```python
from build123d import *

# Parameters (mm, degrees)
SKETCH1_R                                       = 5
SKETCH1_R_2                                     = 1.6
SKETCH1_R_3                                     = 1.25
SKETCH1_R_4                                     = 1.55
BOSS_EXTRUDE1_DEPTH                             = 3.18
CSK_FOR_M2_FLAT_HEAD_MACHINE_SCREW1_D           = 2.4
CSK_FOR_M2_FLAT_HEAD_MACHINE_SCREW1_DEPTH       = 3.508967257
CSK_FOR_M2_FLAT_HEAD_MACHINE_SCREW1_CSINK_D     = 4.4
CSK_FOR_M2_FLAT_HEAD_MACHINE_SCREW1_CSINK_ANGLE = 90
CSK_FOR_M2_FLAT_HEAD_MACHINE_SCREW1_TIP         = 0.721032743
SKETCH3_R                                       = 5
CUT_EXTRUDE4_DEPTH                              = 67.382158748
FILLET2_R                                       = 3
CHAMFER2_SIZE                                   = 1.8


with BuildPart() as part:
    # Sketch1 → Boss-Extrude1 (new body)
    with BuildSketch(Plane(origin=(0, 0, 0), x_dir=(0, 0, -1), z_dir=(1, 0, 0))):
        Polygon((0, 0), (0, 30.2), (2, 32.2), (2, 61.31), (22, 61.31), (22, 41.31), (23.8, 41.31), (23.8, 24.71), (15.9, 24.71), (15.9, 13.26), (13.4, 13.26), (13.4, 11.86), (25.25, 11.86), (25.25, 6.86), (13.4, 6.86), (13.4, 0), align=None)
        with Locations(Location((7, 25.2, 0), (0, 0, 180))):
            Circle(SKETCH1_R, mode=Mode.SUBTRACT)
        with Locations(Location((7, 56.81, 0), (0, 0, 180))):
            Circle(SKETCH1_R_2, mode=Mode.SUBTRACT)
        with Locations(Location((17, 54.81, 0), (0, 0, 180))):
            Circle(SKETCH1_R_2, mode=Mode.SUBTRACT)
        with Locations(Location((22.4, 9.36, 0), (0, 0, 180))):
            Circle(SKETCH1_R_3, mode=Mode.SUBTRACT)
        with Locations(Location((16.4, 9.36, 0), (0, 0, 180))):
            Circle(SKETCH1_R_3, mode=Mode.SUBTRACT)
        with Locations(Location((2.55, 2.55, 0), (0, 0, 180))):
            Circle(SKETCH1_R_4, mode=Mode.SUBTRACT)
        with Locations(Location((2.55, 8.55, 0), (0, 0, 180))):
            Circle(SKETCH1_R_4, mode=Mode.SUBTRACT)
    extrude(amount=BOSS_EXTRUDE1_DEPTH)

    # CSK for M2 Flat Head Machine Screw1
    with Locations(Plane.ZY):
        with Locations((-6.974936087, 46.414674329), (-17.432559713, 42.244769284), (-8.592504199, 35.273154083)):
            CounterSinkHole(CSK_FOR_M2_FLAT_HEAD_MACHINE_SCREW1_D / 2, CSK_FOR_M2_FLAT_HEAD_MACHINE_SCREW1_CSINK_D / 2, depth=CSK_FOR_M2_FLAT_HEAD_MACHINE_SCREW1_DEPTH, counter_sink_angle=CSK_FOR_M2_FLAT_HEAD_MACHINE_SCREW1_CSINK_ANGLE)
            with Locations((0, 0, -(CSK_FOR_M2_FLAT_HEAD_MACHINE_SCREW1_DEPTH + CSK_FOR_M2_FLAT_HEAD_MACHINE_SCREW1_TIP / 2))):  # 118° drill point
                Cone(0, CSK_FOR_M2_FLAT_HEAD_MACHINE_SCREW1_D / 2, CSK_FOR_M2_FLAT_HEAD_MACHINE_SCREW1_TIP, mode=Mode.SUBTRACT)

    # Sketch3 → Cut-Extrude4 (cut, through all)
    with BuildSketch(Plane.ZY):
        with Locations((-11, 41.310865899)):
            Circle(SKETCH3_R)
    extrude(amount=-CUT_EXTRUDE4_DEPTH, mode=Mode.SUBTRACT)

    # Fillet2
    fillet2_edges = [part.edges().sort_by_distance(p)[0] for p in [
        (1.59, 30.2, 0),
        (1.59, 32.2, -2),
    ]]
    fillet(fillet2_edges, radius=FILLET2_R)

    # Chamfer2
    chamfer2_edges = [part.edges().sort_by_distance(p)[0] for p in [
        (1.59, 61.31, -22),
        (1.59, 61.31, -2),
        (1.59, 41.31, -23.8),
    ]]
    chamfer(chamfer2_edges, length=CHAMFER2_SIZE - 0.0001)  # a hair under: the kernel refuses the full size


solid = part.part
```
Model file for the job. Use its own axes, mm. A direction names the side the tool comes from. Give positions to 0.01 mm unless a question says otherwise; leave off trailing zeros. Loops run counter-clockwise (first coordinate to the right, second up) from the corner with the lowest first, then second, coordinate; pieces in that order, holes last. Notation, with made-up numbers: (-8, 48) - (42, 48) arc R10 ccw to (42, 62) - close; hole circle Ø8 at (-26.5, -3). An arc over 180 degrees is marked (long way). One line per item, written item: value. Start each with the question number.
1. Slice it at A-A (y = 2.55). List the corners of the cut face in (x, z).
2. Slice it at B-B (z = -2.55). List the corners of the cut face in (x, y), plus the area to 3 significant figures.
3. Slice it at C-C (x = 1.5). Give the number of separate pieces and of enclosed holes in the cut face, plus the area to 3 significant figures.
4. Which spindle directions (+Z, -Z, +X, -X, +Y, -Y) get a long thin tool onto all of the face, cutting with end or side? Do faces 5 (the flat face through (2, 6.86, -19)), 6 (the flat face through (2, 13.26, -15)), 7 (the flat face through (2, 46, -2)). Say none if no direction does.
5. Slice it at D-D (y = 27.5). List the corners of the cut face in (x, z), plus the area to 3 significant figures.
6. Probe L1, parallel to Z at x = 1.2, y = 9.36; L2, parallel to Z at x = 2.45, y = 54.81; L3, parallel to Y at x = 1.65, z = -2.55. List the from-to ranges inside material, lowest first. Write a range as from..to.
7. Pin check, flat tips, straight feed: pin 1 (1 mm diameter, centred on x = 2, y = 46, fed in from -Z); pin 2 (3 mm diameter, centred on y = 9.36, z = -22.4, fed in from +X); pin 3 (1.6 mm diameter, centred on x = 2, y = 52.5, fed in from +Z); pin 4 (1.6 mm diameter, centred on x = 2, y = 3, fed in from -Z). Stop position of each tip, or through.
8. Pull direction Z, two halves, no side cores. Call faces 1 (the flat face through (2, 51, -22)), 2 (the cylindrical face through (1.57, 23.7, -2.23)), 3 (the flat face through (2, 24.71, -20)), 4 (the cylindrical face through (1.61, 30.09, -0.22)): pulls with the +Z half, pulls with the -Z half, needs draft (parallel to the pull), parting line crosses it, or undercut.
Solution:
1. outline: (0, -13.4) - (3.18, -13.4) - (3.18, -4.1) - (0, -4.1) - close; (0, -1) - (3.18, -1) - (3.18, 0) - (0, 0) - close
2. outline: (0, 0) - (3.18, 0) - (3.18, 1) - (0, 1) - close; (0, 4.1) - (3.18, 4.1) - (3.18, 7) - (0, 7) - close; (0, 10.1) - (3.18, 10.1) - (3.18, 22.92) - (0, 22.92) - close; (0, 27.48) - (3.18, 27.48) - (3.18, 60.06) - (0, 60.06) - close
2. area: 157 mm^2
3. separate pieces: 1
3. enclosed holes: 11
3. area: 977 mm^2
4. face 5: -Z, +X, -X, -Y
4. face 6: -Z, +X, -X
4. face 7: +Z, +X, -X, +Y
5. outline: (0, -23.8) - (3.18, -23.8) - (3.18, -11.44) - (0, -11.44) - close; (0, -2.56) - (3.18, -2.56) - (3.18, 0) - (0, 0) - close
5. area: 47.4 mm^2
6. L1: z = -25.25..-23.65, -21.15..-17.65, -15.15..-3.87, -1.23..0
6. L2: z = -22..-18.6, -15.4..-2
6. L3: y = 0..1, 4.1..7, 10.1..22.92, 27.48..60.06
7. pin 1: stops at z = -22
7. pin 2: stops at x = 3.18
7. pin 3: stops at z = -2
7. pin 4: stops at z = -13.4
8. face 1: pulls with the -Z half
8. face 2: undercut
8. face 3: needs draft
8. face 4: pulls with the +Z half
